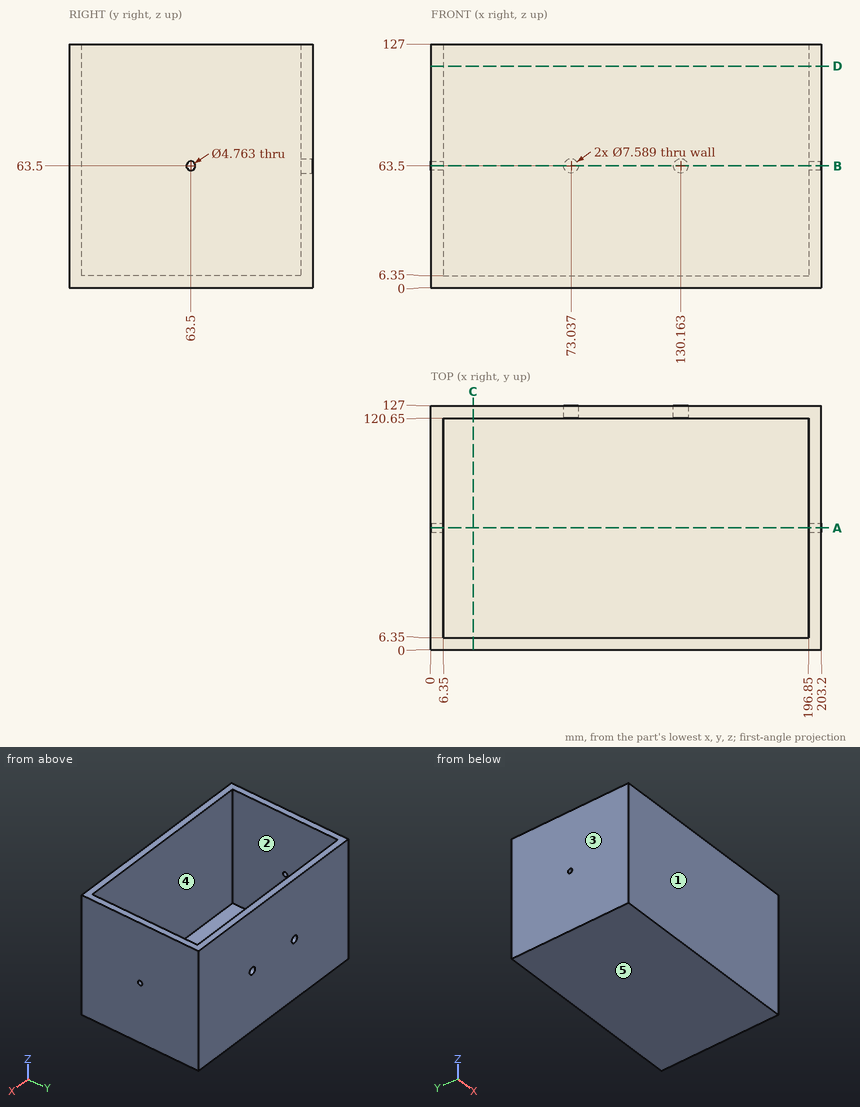
Input: dimensioned drawing with shaded views. Units: mm. Origin: part minimum x, y, z. A direction names the side the tool comes from. Coordinates: 2 decimals unless noted, no trailing zeros. Loops run counter-clockwise (first coordinate to the right, second up) from the corner with the lowest first, then second, coordinate; pieces in that order, holes last. Notation, with made-up numbers: M -0.75,-22 L 57.25,-22 A15 ccw 57.25,-4 Z; hole C 15.5,50 d11. An arc over 180 degrees is marked long. One line per item, written item: value. Start each with the question number.
1) Cut plane D-D (z = 115.5). Return loops of the section in (x, y), then the cut area to 3 significant figures.
2) Reachability of the marked faces 4 and 5 from +Z, -Z, +X, -X, +Y, -Y: full face, straight path, thin tool, end or side. Return the list, or none.
3) Pin query (flat end, axial travel): P1, Ø3, axis at x = 103, y = 89.5, coming from the +Z side; P2, Ø7, axis at x = 130.16, z = 63.5, coming from the +Y side; P3, Ø4, axis at x = 43, z = 83, coming from the -Y side; P4, Ø4.5, axis at y = 63.5, z = 63.5, coming from the +X side. Return the tip coordinate at first contact, or that it passes through.
4) Cut plane C-C (x = 22). Return loops of the section in (y, z), then the cut area to 3 significant figures.
5) Draft query along Y for the marked faces 1, 2 and 3. Return one class per face: released by +Y, released by -Y, zero draft, split by the parting line, or undercut.
6) Cut plane A-A (y = 63.5). Return loops of the section in (x, z), then the cut area to 3 significant figures.
7) Cut plane B-B (z = 63.5). Return loops of the section in (x, y).
8) Material intervals for L1, parallel to X at y = 97, z = 69; L2, parallel to Y at x = 181.5, z = 114.5, sorted ascending. Write a range as from..to.
Evaluation:
1. outline: M 0,0 L 203.2,0 L 203.2,127 L 0,127 Z; hole M 6.35,6.35 L 196.85,6.35 L 196.85,120.65 L 6.35,120.65 Z
1. area: 4,030 mm^2
2. face 4: +Z
2. face 5: -Z, +X, -X, +Y, -Y
3. P1: z = 6.35
3. P2: y = 6.35
3. P3: y = 0
3. P4: through
4. outline: M 0,0 L 127,0 L 127,127 L 120.65,127 L 120.65,6.35 L 6.35,6.35 L 6.35,127 L 0,127 Z
4. area: 2,340 mm^2
5. face 1: released by -Y
5. face 2: undercut
5. face 3: zero draft
6. outline: M 0,0 L 203.2,0 L 203.2,61.12 L 196.85,61.12 L 196.85,6.35 L 6.35,6.35 L 6.35,61.12 L 0,61.12 Z; M 0,65.88 L 6.35,65.88 L 6.35,127 L 0,127 Z; M 196.85,65.88 L 203.2,65.88 L 203.2,127 L 196.85,127 Z
6. area: 2,760 mm^2
7. outline: M 0,0 L 203.2,0 L 203.2,61.12 L 196.85,61.12 L 196.85,6.35 L 6.35,6.35 L 6.35,61.12 L 0,61.12 Z; M 0,65.88 L 6.35,65.88 L 6.35,120.65 L 69.24,120.65 L 69.24,127 L 0,127 Z; M 76.83,120.65 L 126.37,120.65 L 126.37,127 L 76.83,127 Z; M 133.96,120.65 L 196.85,120.65 L 196.85,65.88 L 203.2,65.88 L 203.2,127 L 133.96,127 Z
8. L1: 0..6.35, 196.85..203.2
8. L2: 0..6.35, 120.65..127
